```python
from build123d import *


with BuildPart() as f1:
    # F0 (on Front) → F1 (revolve)
    with BuildSketch(Plane.XZ):
        with BuildLine():
            Line((-5.512861, 50.567072), (-12.721327, 50.440166))
            Line((-12.721327, 50.440166), (-12.721327, -45.461077))
            Line((-12.721327, -45.461077), (-10.906334, -52.084621))
            Line((-10.906334, -52.084621), (-9.713333, -51.757713))
            Line((-9.713333, -51.757713), (-5.205728, -47.478069))
            Line((-5.205728, -47.478069), (-5.205728, -37.064623))
            Line((-5.205728, -37.064623), (-8.348268, -24.129307))
            ThreePointArc((-8.348268, -24.129307), (-9.293465, -19.217544), (-9.76137, -14.237597))
            Line((-9.76137, -14.237597), (-9.76137, 14.535546))
            Line((-9.76137, 14.535546), (-7.231527, 38.962592))
            ThreePointArc((-7.231527, 38.962592), (-5.927004, 40.733404), (-3.833717, 41.408464))
            Line((-3.833717, 41.408464), (13.918695, 41.408464))
            Line((13.918695, 41.408464), (13.918695, 48.971001))
            Line((13.918695, 48.971001), (-5.512861, 48.971001))
            Line((-5.512861, 48.971001), (-5.512861, 50.567072))
        make_face()
    revolve(axis=Axis((-18.336685, 0, -7.719919), (0, 0, -1)))


solid = f1.part
```
Geometry: final body of the model. Coordinates: model frame, mm. A direction names the side the tool comes from. Round coordinates to 2 decimals unless told otherwise and drop trailing zeros. Order: outer loops, then holes, each group sorted by start corner. A loop starts at its lowest first (then second) coordinate and runs counter-clockwise, first axis right, second up. Notation, with made-up numbers: (13, 41) -> (32, 41) arc R24 ccw to (32, 77) -> close; hole circle Ø4 at (-1, -33.5). An arc over 180 degrees is marked (long way). Use one line per item in the form item = value. Start each with the question number.
1. Reachability of faces 4 (the face through (-24.296, -0.262, 50.446)), 5 (the face through (-6.207, 5.029, -42.198)), 6 (the face through (-26.16, 6, 26.92)) from +Z, -Z, +X, -X, +Y, -Y: full face, straight path, thin tool, end or side. Return the list, or none.
2. Draft query along X for faces 1 (the face through (-23.947, -0.247, 1.818)), 2 (the face through (-6.105, -3.852, 49.78)), 3 (the face through (-32, 7, 41.408)). Return one class per face: pulls with the +X half, pulls with the -X half, needs draft (parallel to the pull), parting line crosses it, or undercut.
3. Pin query (flat end, axial travel): pin 1 Ø2 at (x, z) = (-18.5, -6) entering from -Y; pin 2 Ø1.5 at (x, z) = (-8.5, 38.5) entering from -Y; pin 3 Ø12 at (x, y) = (-5.5, -21.5) entering from +Z; pin 4 Ø4 at (y, z) = (14.5, -31.5) entering from -X. Return the tip coordinate at first contact, or that it passes through.
4. Line query: probe 1 along X at (y, z) = (0, -5); probe 2 along Z at (x, y) = (-17, -18); probe 3 along X at (y, z) = (-2, -24). Output: solid intervals per line, ascending.
5. Cut plane C-C (y = 17.5). Return the cut outline in (x, z), then the cut area to 3 significant figures.
6. Cut plane B-B (z = 5). Return the cut outline in (x, y).
7. Cut plane D-D (x = 10). Return the cut outline in (y, z), then the cut area to 3 significant figures.
Solution:
q1.face_4 = +Z
q1.face_5 = -Z
q1.face_6 = none
q2.face_1 = undercut
q2.face_2 = parting line crosses it
q2.face_3 = needs draft
q3.pin_1 = -8.58
q3.pin_2 = -6.31
q3.pin_3 = 48.97
q3.pin_4 = through
q4.probe_1 = -26.91 to -23.95, -12.72 to -9.76
q4.probe_2 = 41.41 to 48.97
q4.probe_3 = -28.09 to -23.58, -13.09 to -8.58
q5.outline = (-45.43, 41.41) -> (8.76, 41.41) -> (8.76, 48.97) -> (-45.43, 48.97) -> close
q5.area = 410 mm^2
q6.outline = circle Ø17.15 at (-18.34, 0); hole circle Ø11.23 at (-18.34, 0)
q7.outline = (-15.41, 41.41) -> (15.41, 41.41) -> (15.41, 48.97) -> (-15.41, 48.97) -> close
q7.area = 233 mm^2
